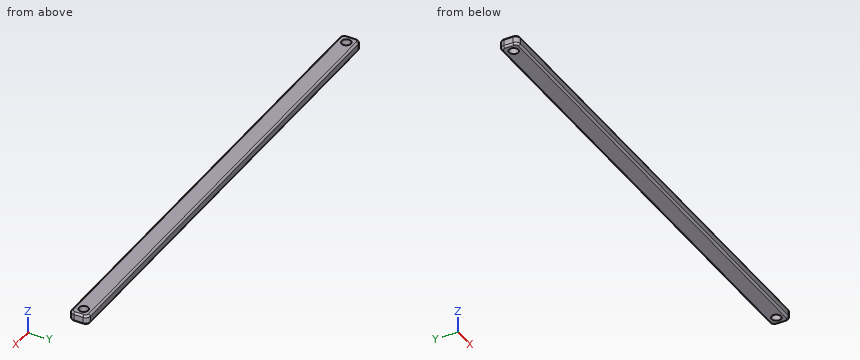
```python
from build123d import *

# Parameters (mm, degrees)
F0_R     = 12.7
F1_DEPTH = 25.4
F3_D     = 25.4
F4_R     = 5.08


with BuildPart() as f1:
    # F0 (on Top) → F1 (new body)
    with BuildSketch(Plane.XY):
        with BuildLine():
            Line((769.519733, 50.8), (-538.580267, 50.8))
            ThreePointArc((-538.580267, 50.8), (-547.560523, 47.080256), (-551.280267, 38.1))
            Line((-551.280267, 38.1), (-551.280267, 12.7))
            ThreePointArc((-551.280267, 12.7), (-547.560523, 3.719744), (-538.580267, 0))
            Line((-538.580267, 0), (769.519733, 0))
            ThreePointArc((769.519733, 0), (778.499989, 3.719744), (782.219733, 12.7))
            Line((782.219733, 12.7), (782.219733, 38.1))
            ThreePointArc((782.219733, 38.1), (778.499989, 47.080256), (769.519733, 50.8))
        make_face()
        with Locations((-525.880267, 25.4)):
            Circle(F0_R, mode=Mode.SUBTRACT)
    extrude(amount=F1_DEPTH)

    # F3 (through all)
    with Locations(Plane(origin=(0, 0, 0), x_dir=(1, 0, 0), z_dir=(0, 0, -1))):
        with Locations((756.819733, -25.4)):
            Hole(F3_D / 2)

    # F4
    f4_edges = [f1.edges().sort_by_distance(p)[0] for p in [
        (115.469733, 0, 0),
        (-551.280267, 25.4, 0),
        (115.469733, 50.8, 0),
        (782.219733, 25.4, 0),
        (115.469733, 0, 25.4),
        (782.219733, 25.4, 25.4),
        (115.469733, 50.8, 25.4),
        (-551.280267, 25.4, 25.4),
    ]]
    fillet(f4_edges, radius=F4_R)


solid = f1.part
```
Model file for the job. Use its own axes, mm. Round coordinates to 2 decimals unless told otherwise and drop trailing zeros. Write each loop counter-clockwise with the first axis right and the second up, starting at its lowest first coordinate (ties: lowest second). Pieces come first, ordered by that corner, then holes. Notation, with made-up numbers: M 65,14.25 L 74,14.25 A21 cw 74,26.25 Z; hole C -13.75,11 d9. An arc over 180 degrees is marked long. Put each result on its own line as item: value.
Item 1: Probe L1, parallel to X at y = 18, z = 9.5; L2, parallel to X at y = 17, z = 11; L3, parallel to Y at x = 559, z = 3.75. List the from-to ranges inside material, lowest first. Write a range as from..to.
Responses:
L1: -551.28..-536.2, -515.56..746.5, 767.14..782.22
L2: -551.28..-535.41, -516.36..747.29, 766.34..782.22
L3: 0.18..50.62
Item 2: Cut at B-B (y = 25.4). List the corners of the cut face in (x, z).
Responses:
outline: M -551.28,5.08 A5.08 ccw -546.2,0 L -538.58,0 L -538.58,25.4 L -546.2,25.4 A5.08 ccw -551.28,20.32 Z; M -513.18,0 L 744.12,0 L 744.12,25.4 L -513.18,25.4 Z; M 769.52,0 L 777.14,0 A5.08 ccw 782.22,5.08 L 782.22,20.32 A5.08 ccw 777.14,25.4 L 769.52,25.4 Z
Item 3: Cut at A-A (z = 15). List the corners of the cut face in (x, y), and give its area (3 significant figures).
Responses:
outline: M -551.28,12.7 A12.7 ccw -538.58,0 L 769.52,0 A12.7 ccw 782.22,12.7 L 782.22,38.1 A12.7 ccw 769.52,50.8 L -538.58,50.8 A12.7 ccw -551.28,38.1 Z; hole C -525.88,25.4 d25.4; hole C 756.82,25.4 d25.4
area: 66,600 mm²
Item 4: Cut at C-C (x = 411.5). List the corners of the cut face in (y, z).
Responses:
outline: M 0,5.08 A5.08 ccw 5.08,0 L 45.72,0 A5.08 ccw 50.8,5.08 L 50.8,20.32 A5.08 ccw 45.72,25.4 L 5.08,25.4 A5.08 ccw 0,20.32 Z
Item 5: Flat gauge pins, fed straight in: P1, Ø8, axis at y = 45.5, z = 10.5, coming from the -X side; P2, Ø12, axis at x = 120, y = 19.5, coming from the -Z side. Where does each tip first touch, or does it go through?
Responses:
P1: x = -550.82
P2: z = 0
